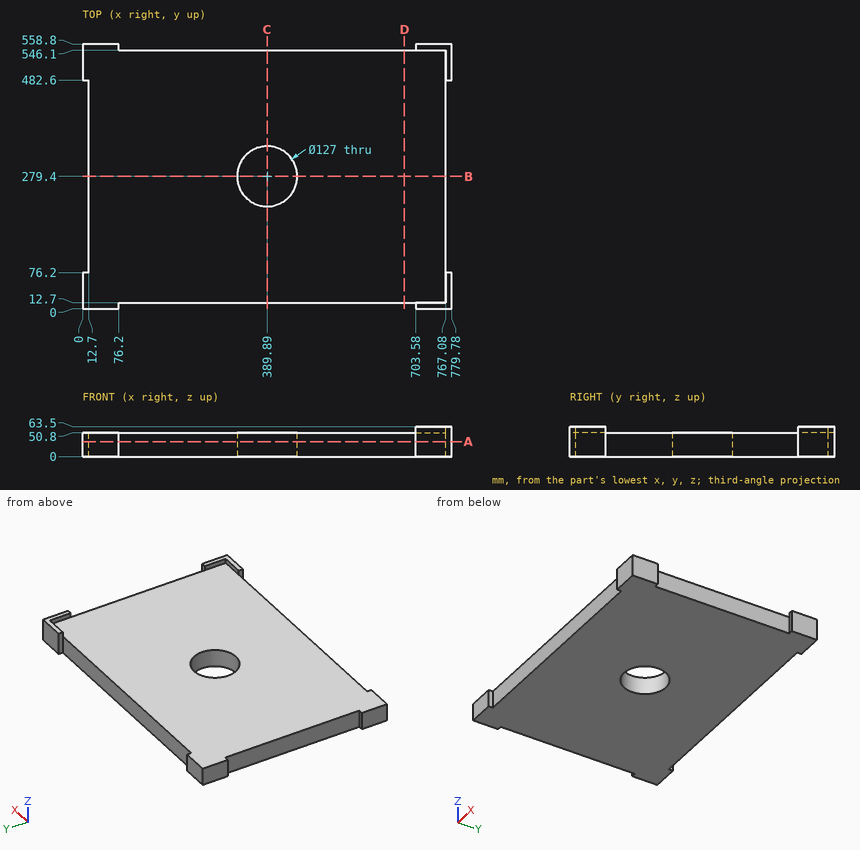
Part print with two shaded views. Sizes in mm from the minimum x, y, z corner. Round coordinates to 2 decimals unless told otherwise and drop trailing zeros. Order: outer loops, then holes, each group sorted by start corner. A loop starts at its lowest first (then second) coordinate and runs counter-clockwise, first axis right, second up. Notation, with made-up numbers: M -6,8.25 L 9,8.25 A26 cw 9,25.25 Z; hole C 38.5,26.25 d2. An arc over 180 degrees is marked long. Put each result on its own line as item: value. Start each with the question number.
1. Slice it at B-B on y = 279.4. List the corners of the cut face in (x, z).
2. Slice it at D-D on x = 679.5. List the corners of the cut face in (y, z).
3. Slice it at C-C on x = 389.89. List the corners of the cut face in (y, z).
4. Slice it at A-A on z = 32. List the corners of the cut face in (x, y), then the cut area to 3 significant figures.
5. Drill centre lines: probe 1 along X at (y, z) = (279, 31); probe 2 along Y at (x, z) = (389, 16); probe 3 along Z at (x, y) = (145, 179). Where is each one in solid material? Low to high. Write a range as [from, to].
6. Drop flat-ended pins along their axis: pin 1 (10 mm diameter, centred on x = 560.5, z = 28, fed in from -Y); pin 2 (1.5 mm diameter, centred on x = 599, y = 82, fed in from -Z); pin 3 (6.5 mm diameter, centred on y = 45.5, z = 54.5, fed in from -X); pin 4 (8 mm diameter, centred on y = 165, z = 30.5, fed in from -X). Give the stop position or say it passes through.
Findings:
1. outline: M 12.7,0 L 326.39,0 L 326.39,50.8 L 12.7,50.8 Z; M 453.39,0 L 767.08,0 L 767.08,50.8 L 453.39,50.8 Z
2. outline: M 12.7,0 L 546.1,0 L 546.1,50.8 L 12.7,50.8 Z
3. outline: M 12.7,0 L 215.9,0 L 215.9,50.8 L 12.7,50.8 Z; M 342.9,0 L 546.1,0 L 546.1,50.8 L 342.9,50.8 Z
4. outline: M 0,0 L 76.2,0 L 76.2,12.7 L 703.58,12.7 L 703.58,0 L 779.78,0 L 779.78,76.2 L 767.08,76.2 L 767.08,482.6 L 779.78,482.6 L 779.78,558.8 L 703.58,558.8 L 703.58,546.1 L 76.2,546.1 L 76.2,558.8 L 0,558.8 L 0,482.6 L 12.7,482.6 L 12.7,76.2 L 0,76.2 Z; hole C 389.89,279.4 d127
4. area: 397,000 mm2
5. probe 1: [12.7, 326.39], [453.39, 767.08]
5. probe 2: [12.7, 215.91], [342.89, 546.1]
5. probe 3: [0, 50.8]
6. pin 1: y = 12.7
6. pin 2: z = 0
6. pin 3: x = 767.08
6. pin 4: x = 12.7
